Study the drawing (mm; zero at the part's minimum x, y, z) and answer. Give positions to 0.01 mm unless a question says otherwise; leave off trailing zeros. Order: outer loops, then holes, each group sorted by start corner. A loop starts at its lowest first (then second) coordinate and runs counter-clockwise, first axis right, second up. Notation, with made-up numbers: (-1, -12.75) - (58, -12.75) arc R5 ccw to (58, -8.75) - close; hole circle Ø7 at (9, 10.5). An arc over 180 degrees is marked (long way). Return JSON: item names as keys, results as strings.
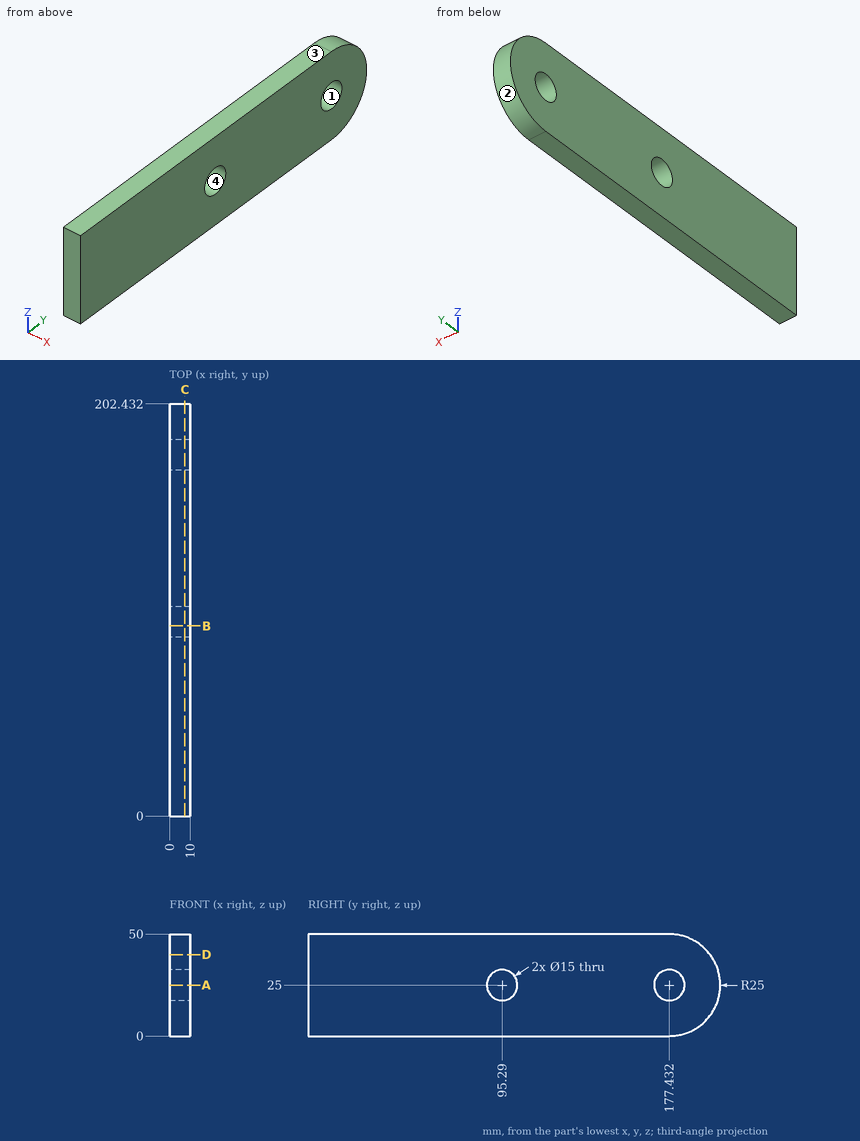
Q1. A cutting plane is placed at A-A (z = 25). Write down the section's boundary in (x, y).
Values:
{"outline": "(0, 0) - (10, 0) - (10, 87.79) - (0, 87.79) - close; (0, 102.79) - (10, 102.79) - (10, 169.93) - (0, 169.93) - close; (0, 184.93) - (10, 184.93) - (10, 202.43) - (0, 202.43) - close"}
Q2. A cutting plane is placed at C-C (x = 7.5). Write down the section's boundary in (y, z), and give its area (3 significant figures).
Values:
{"outline": "(0, 0) - (177.43, 0) arc R25 ccw to (177.43, 50) - (0, 50) - close; hole circle Ø15 at (95.29, 25); hole circle Ø15 at (177.43, 25)", "area": "9,500 mm²"}
Q3. Consider L1, parallel to Y at x = 2.5, z = 25; L2, parallel to Y at x = 9.5, z = 22 (1 decimal); L3, parallel to Z at x = 6.75, y = 96.5. Determine where each line is inside the solid, lowest interval first.
Values:
{"L1": "y = 0 to 87.79, 102.79 to 169.93, 184.93 to 202.43", "L2": "y = 0 to 88.4, 102.2 to 170.6, 184.3 to 202.3", "L3": "z = 0 to 17.6, 32.4 to 50"}
Q4. Determine the mould class of the marked faces 1, 2, 3 and 4 for opening direction Z: released by +Z, released by -Z, zero draft, split by the parting line, or undercut.
Values:
{"face 1": "undercut", "face 2": "split by the parting line", "face 3": "released by +Z", "face 4": "undercut"}
Q5. Given pin 1 (3 mm diameter, centred on y = 31.5, z = 42, fed in from -X); pin 2 (4 mm diameter, centred on x = 8.5, z = 21.5, fed in from +Y), each flat-ended and moving along its own axis, determine where each tip first touches the part or whether it passes through.
Values:
{"pin 1": "stops at x = 0", "pin 2": "stops at y = 202.39"}
Q6. A cutting plane is placed at B-B (y = 93.5). Write down the section's boundary in (x, z).
Values:
{"outline": "(0, 0) - (10, 0) - (10, 17.72) - (0, 17.72) - close; (0, 32.28) - (10, 32.28) - (10, 50) - (0, 50) - close"}
Q7. A cutting plane is placed at D-D (z = 40). Write down the section's boundary in (x, y), and give its area (3 significant figures).
Values:
{"outline": "(0, 0) - (10, 0) - (10, 197.43) - (0, 197.43) - close", "area": "1,970 mm²"}
